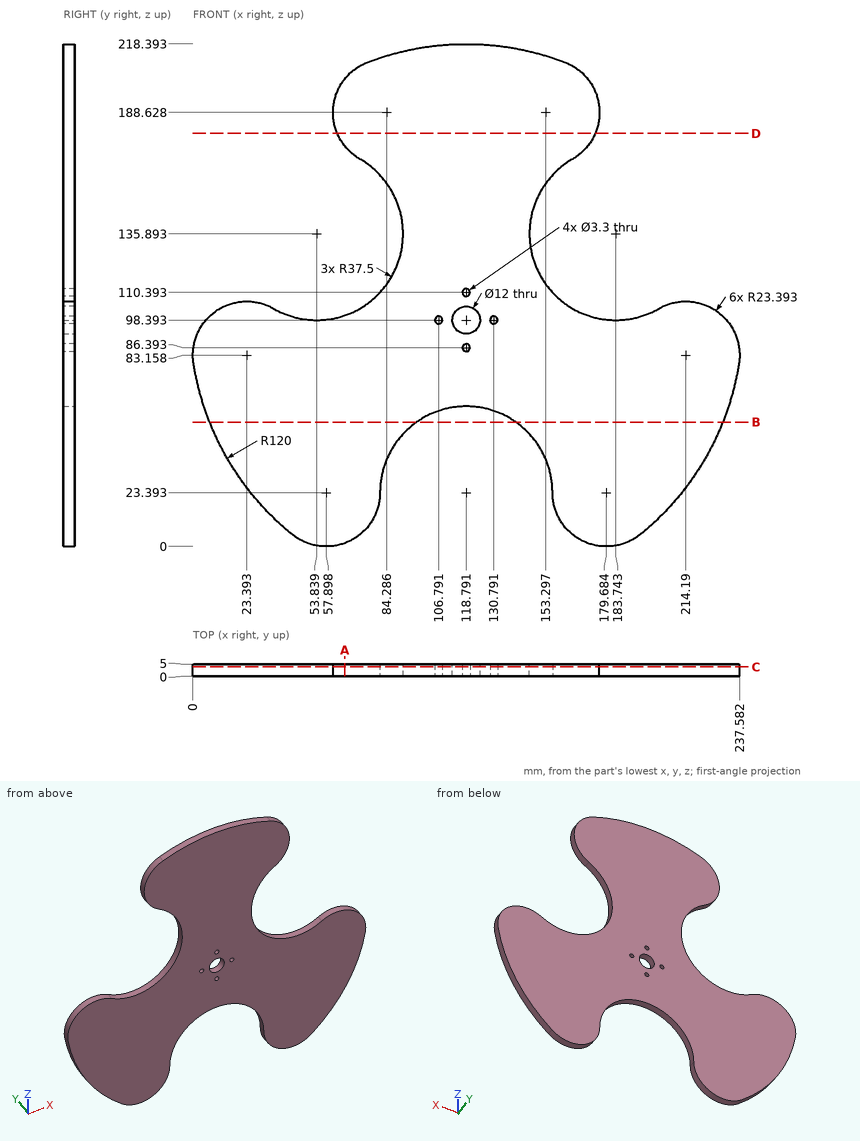
Geometry: see drawing. Coordinates: mm, zero at the bounding-box minimum. Coordinates: 2 decimals unless noted, no trailing zeros. Write each loop counter-clockwise with the first axis right and the second up, starting at its lowest first coordinate (ties: lowest second). Pieces come first, ordered by that corner, then holes.
1) Section D-D on z = 179.5. Output: boundary loops of the cut face in (x, y) (1 decimal).
2) Section B-B on z = 54. Output: boundary loops of the cut face in (x, y) (1 decimal).
3) Pin query (flat end, axial travel): pin 1 Ø7 at (x, z) = (118.79, 98.39) entering from +Y; pin 2 Ø3 at (x, y) = (162, 3) entering from -Z; pin 3 Ø3 at (x, y) = (182, 4) entering from +Z. Return the tip coordinate at first contact, or that it passes through.
4) Material intervals for line 1 along Z through (x, y) = (162.5, 0.7) (1 decimal); line 2 along X through (y, z) = (2.85, 20.5) (1 decimal); line 3 along X through (y, z) = (1.5, 79.5) (1 decimal), sorted ascending.
5) Section A-A on x = 66. Output: boundary loops of the cut face in (y, z).
6) Section C-C on y = 3.95. State how many separate pieces and enclosed holes the cut face has, and give its area (3 significant figures).
Check result:
1. outline: (62.7, 0) - (174.8, 0) - (174.8, 5) - (62.7, 5) - close
2. outline: (7.3, 0) - (97.1, 0) - (97.1, 5) - (7.3, 5) - close; (140.5, 0) - (230.3, 0) - (230.3, 5) - (140.5, 5) - close
3. pin 1: passes through
3. pin 2: stops at z = 6.5
3. pin 3: stops at z = 98.53
4. line 1: z = 7.5 to 105, 166.8 to 210.1
4. line 2: x = 27.5 to 81.1, 156.5 to 210.1
4. line 3: x = 0.3 to 237.3
5. outline: (0, 1.45) - (5, 1.45) - (5, 100.42) - (0, 100.42) - close; (0, 174.04) - (5, 174.04) - (5, 203.22) - (0, 203.22) - close
6. separate pieces: 1
6. enclosed holes: 5
6. area: 26,400 mm2
